Answer from the drawing. Dimensions are ordinates in mm from the lowest x, y and z of the part. A direction names the side the tool comes from. Round coordinates to 2 decimals unless told otherwise and drop trailing zeros. Write each loop counter-clockwise with the first axis right and the second up, starting at its lowest first coordinate (ties: lowest second). Pieces come first, ordered by that corner, then holes. Notation, with made-up numbers: (80.5, 52.5) - (128.5, 52.5) arc R20 cw to (128.5, 80.5) - close; hole circle Ø1 at (64.25, 3.25). An arc over 180 degrees is marked (long way). Write item = value, one per line. Start each with the question number.
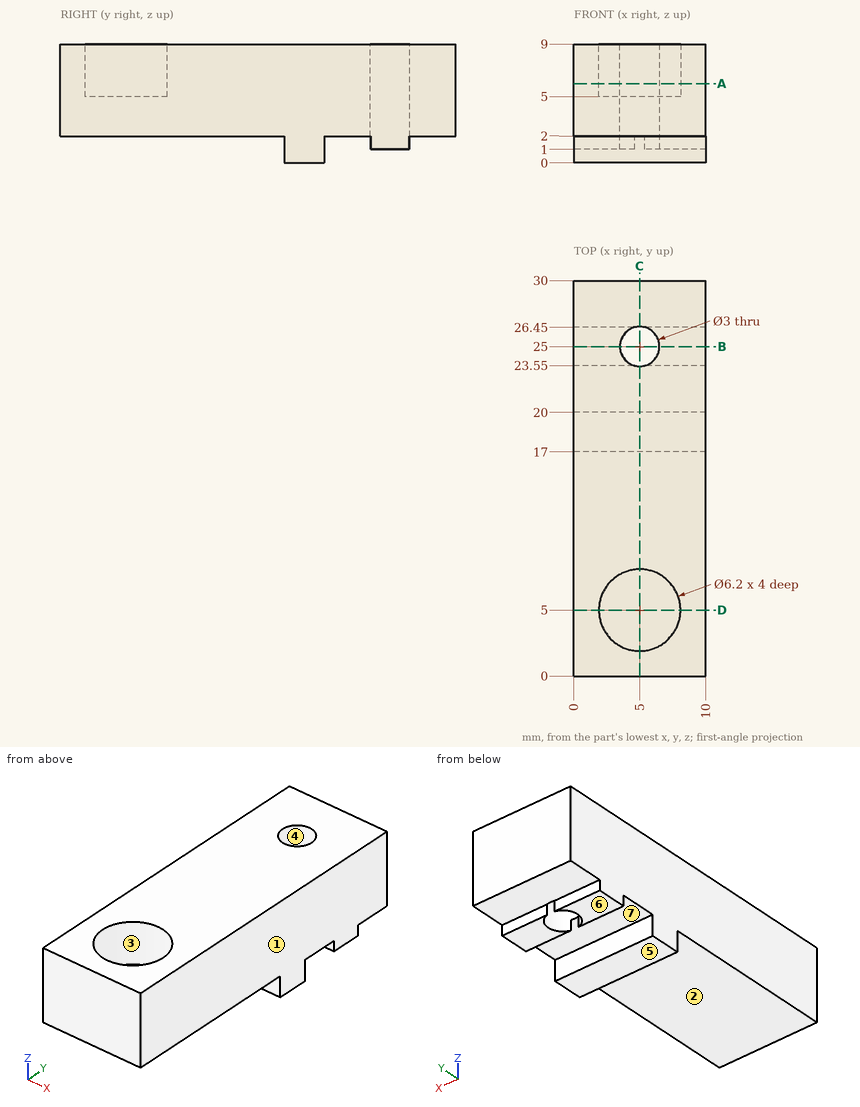
1. Find section B-B on y = 25. Give the vertices of the cut face in (x, z), plus the area to 3 significant figures.
2. Which of the six approach directions +Z, -Z, +X, -X, +Y, -Y give full straight-line access (tool end or side, diameter ignored) to the marked faces 5, 6 and 7?
3. For a pull along X with two mould halves and no side action, classify the marked faces 1, 2, 3 and 4 as released by +X, released by -X, zero draft, split by the parting line, or undercut.
4. Consider line 1 (Y direction, x = 5, z = 7); line 2 (Y direction, x = 5, z = 4.25); line 3 (X direction, y = 25, z = 6.5). Determine where each line is inside the solid, lowest interval first.
5. Each of these flat-tipped pins is pushed along its axis until it touches: pin 1 (1.1 mm diameter, centred on x = 5.5, y = 27.5, fed in from -Z); pin 2 (5 mm diameter, centred on x = 5, y = 5, fed in from +Z); pin 3 (0.5 mm diameter, centred on x = 3, z = 1.5, fed in from -Y). Where does it stop, or does it pass through?
6. Find section A-A on z = 6. Give the vertices of the cut face in (x, y), plus the area to 3 significant figures.
7. Find section D-D on y = 5. Give the vertices of the cut face in (x, z), plus the area to 3 significant figures.
8. Find section C-C on x = 5. Give the vertices of the cut face in (y, z).
Answer key:
q1.outline = (0, 1) - (3.5, 1) - (3.5, 9) - (0, 9) - close; (6.5, 1) - (10, 1) - (10, 9) - (6.5, 9) - close
q1.area = 56.0 mm²
q2.face_5 = -Z, +X, -X, +Y, -Y
q2.face_6 = -Z, +X, -X, +Y
q2.face_7 = -Z, +X, -X
q3.face_1 = released by +X
q3.face_2 = zero draft
q3.face_3 = undercut
q3.face_4 = undercut
q4.line_1 = 0 to 1.9, 8.1 to 23.5, 26.5 to 30
q4.line_2 = 0 to 23.5, 26.5 to 30
q4.line_3 = 0 to 3.5, 6.5 to 10
q5.pin_1 = 2
q5.pin_2 = 5
q5.pin_3 = 17
q6.outline = (0, 0) - (10, 0) - (10, 30) - (0, 30) - close; hole circle Ø6.2 at (5, 5); hole circle Ø3 at (5, 25)
q6.area = 263 mm²
q7.outline = (0, 2) - (10, 2) - (10, 9) - (8.1, 9) - (8.1, 5) - (1.9, 5) - (1.9, 9) - (0, 9) - close
q7.area = 45.2 mm²
q8.outline = (0, 2) - (17, 2) - (17, 0) - (20, 0) - (20, 2) - (23.5, 2) - (23.5, 9) - (8.1, 9) - (8.1, 5) - (1.9, 5) - (1.9, 9) - (0, 9) - close; (26.5, 2) - (30, 2) - (30, 9) - (26.5, 9) - close
